CAD build for the part. Positions are in the model's coordinates, mm. A direction names the side the tool comes from. Round coordinates to 2 decimals unless told otherwise and drop trailing zeros. Order: outer loops, then holes, each group sorted by start corner. A loop starts at its lowest first (then second) coordinate and runs counter-clockwise, first axis right, second up. Notation, with made-up numbers: (52, 49.25) -> (71, 49.25) arc R24 ccw to (71, 64.25) -> close; hole circle Ø1 at (-29, -4). An arc over 180 degrees is marked (long way). Return JSON: item names as keys, results as strings. Group by question number.
Q1. Cut at C-C (z = -3). Write the cut outline in (x, y), then the cut area to 3 significant figures.
Q2. Probe line 1 along X through (y, z) = (-1.25, -31.5); line 2 along Y through (x, z) = (13.5, -43); line 3 along Z through (x, y) = (82, -0.5). List the from-to ranges inside material, lowest first.
Q3. Cut at D-D (x = 38). Write the cut outline in (y, z), then the cut area to 3 significant figures.
Q4. Flat gauge pins, fed straight in: pin 1 (12 mm diameter, centred on x = 76.5, z = -30.5, fed in from -Y); pin 2 (0.8 mm diameter, centred on y = -1.5, z = -51.5, fed in from -X); pin 3 (4 mm diameter, centred on x = 63.5, z = -8, fed in from -Y). Where does each tip first touch, or does it go through?
Q5. Cut at A-A (y = -1). Write the cut outline in (x, z), then the cut area to 4 significant figures.
Q6. Which spindle directions (+Z, -Z, +X, -X, +Y, -Y) get a long thin tool onto all of the face, cutting with end or side? Do faces 1 (the flat face through (28.45, -1, -3)), 2 (the flat face through (61.6, -1, -52)), 3 (the flat face through (60, -1, -4.5)), 4 (the flat face through (54, -1, -53.2)). Say none if no direction does.
Q7. Cut at B-B (x = 72). Write the cut outline in (y, z).
from build123d import *

# Parameters (mm, degrees)
SKETCH1_W           = 85.6
SKETCH1_H           = 55.7
BOSS_EXTRUDE1_DEPTH = 7.1
SKETCH2_W           = 20.3
SKETCH2_H           = 2.5
SKETCH2_W_2         = 15.3
BOSS_EXTRUDE2_DEPTH = 2.5
SKETCH3_W           = 15
SKETCH3_H           = 14.9
BOSS_EXTRUDE3_DEPTH = 2


with BuildPart() as part:
    # Sketch1 → Boss-Extrude1 (new body)
    with BuildSketch(Plane(origin=(0, 0, 0), x_dir=(1, 0, 0), z_dir=(0, 1, 0))):
        with Locations((42.8, 27.85)):
            Rectangle(SKETCH1_W, SKETCH1_H)
    extrude(amount=BOSS_EXTRUDE1_DEPTH)

    # Sketch2 → Boss-Extrude2 (add)
    with BuildSketch(Plane.XZ):
        with Locations((38.6, -3.25)):
            Rectangle(SKETCH2_W, SKETCH2_H)
        with Locations((60.45, -3.25)):
            Rectangle(SKETCH2_W, SKETCH2_H)
        with Locations((53.95, -51.95)):
            Rectangle(SKETCH2_W_2, SKETCH2_H)
        with Locations((36.1, -51.95)):
            Rectangle(SKETCH2_W_2, SKETCH2_H)
    extrude(amount=BOSS_EXTRUDE2_DEPTH)

    # Sketch3 → Boss-Extrude3 (add)
    with BuildSketch(Plane.XZ):
        with Locations((77.1, -32.75)):
            Rectangle(SKETCH3_W, SKETCH3_H)
    extrude(amount=BOSS_EXTRUDE3_DEPTH)


solid = part.part
Solution:
{
 "1": {"outline": "(0, 0) -> (28.45, 0) -> (28.45, -2.5) -> (48.75, -2.5) -> (48.75, 0) -> (50.3, 0) -> (50.3, -2.5) -> (70.6, -2.5) -> (70.6, 0) -> (85.6, 0) -> (85.6, 7.1) -> (0, 7.1) -> close", "area": "709 mm²"},
 "2": {"line 1": "x = 69.6 to 84.6", "line 2": "y = 0 to 7.1", "line 3": "z = -40.2 to -25.3"},
 "3": {"outline": "(-2.5, -53.2) -> (0, -53.2) -> (0, -55.7) -> (7.1, -55.7) -> (7.1, 0) -> (0, 0) -> (0, -2) -> (-2.5, -2) -> (-2.5, -4.5) -> (0, -4.5) -> (0, -50.7) -> (-2.5, -50.7) -> close", "area": "408 mm²"},
 "4": {"pin 1": "stops at y = -2", "pin 2": "stops at x = 28.45", "pin 3": "stops at y = 0"},
 "5": {"outline": "(28.45, -53.2) -> (43.75, -53.2) -> (43.75, -50.7) -> (28.45, -50.7) -> close; (28.45, -4.5) -> (48.75, -4.5) -> (48.75, -2) -> (28.45, -2) -> close; (46.3, -53.2) -> (61.6, -53.2) -> (61.6, -50.7) -> (46.3, -50.7) -> close; (50.3, -4.5) -> (70.6, -4.5) -> (70.6, -2) -> (50.3, -2) -> close; (69.6, -40.2) -> (84.6, -40.2) -> (84.6, -25.3) -> (69.6, -25.3) -> close", "area": "401.5 mm²"},
 "6": {"face 1": "+Z, -Z, -X, -Y", "face 2": "-Z, +X, -Y", "face 3": "+X, -X, -Y", "face 4": "-Z, +X, -X, -Y"},
 "7": {"outline": "(-2, -40.2) -> (0, -40.2) -> (0, -55.7) -> (7.1, -55.7) -> (7.1, 0) -> (0, 0) -> (0, -25.3) -> (-2, -25.3) -> close"}
}
